Verification items for the finished model (mm, model axes). Coordinates: 2 decimals unless noted, no trailing zeros. Write each loop counter-clockwise with the first axis right and the second up, starting at its lowest first coordinate (ties: lowest second). Pieces come first, ordered by that corner, then holes. Notation, with made-up numbers: M 60.25,0.5 L 81.25,0.5 A12 ccw 81.25,19.5 Z; hole C 79.25,35.5 d11. An arc over 180 degrees is marked long. Answer in a Markdown table with one row per item.
Autodesk Fusion 360 part; units mm, degrees
sketch "スケッチ1" plane through (0, 0, 0) normal (0, 1, 0) x (1, 0, 0)
  line L0 (-132, 0) -> (132, 0)
  line L1 (-132, 0) -> (-132, -10)
  line L2 (-132, -10) -> (-128, -10)
  line L3 (-128, -10) -> (-128, -20)
  line L4 (-128, -20) -> (-132, -20)
  line L5 (-132, -20) -> (-132, -30)
  line L6 (-132, -30) -> (-128, -30)
  line L7 (-128, -30) -> (-128, -40)
  line L8 (-128, -40) -> (-132, -40)
  line L9 (-132, -40) -> (-132, -50)
  line L10 (-132, -50) -> (-77, -50)
  line L11 (-77, -50) -> (-77, -42)
  line L12 (132, 0) -> (132, -10)
  line L13 (132, -10) -> (128, -10)
  line L14 (128, -10) -> (128, -20)
  line L15 (128, -20) -> (132, -20)
  line L16 (132, -20) -> (132, -30)
  line L17 (132, -30) -> (128, -30)
  line L18 (128, -30) -> (128, -40)
  line L19 (128, -40) -> (132, -40)
  line L20 (132, -40) -> (132, -50)
  line L21 (132, -50) -> (72, -50)
  line L22 (72, -50) -> (72, -42)
  line L23 (-77, -42) -> (-65, -42)
  line L24 (-65, -42) -> (-65, -50)
  line L25 (-37, -50) -> (60, -50)
  line L26 (60, -50) -> (60, -42)
  line L27 (60, -42) -> (72, -42)
  line L28 (-113, -50) -> (-97, -50)
  line L29 (-97, -50) -> (-97, -55)
  line L30 (-97, -55) -> (-113, -55)
  line L31 (-113, -55) -> (-113, -50)
  line L32 (97, -50) -> (113, -50)
  line L33 (113, -50) -> (113, -55)
  line L34 (113, -55) -> (97, -55)
  line L35 (97, -55) -> (97, -50)
  line L36 (-38, 0) -> (38, 0)
  line L37 (38, 0) -> (38, -12)
  line L38 (38, -12) -> (-38, -12)
  line L39 (-38, -12) -> (-38, 0)
  line L40 (-37, -50) -> (-37, -42)
  line L41 (-37, -42) -> (-55, -42)
  line L42 (-55, -42) -> (-55, -50)
  line L43 (-55, -50) -> (-65, -50)
  point P0 (0, -20)
  point P1 (-105, -50)
  point P2 (105, -50)
  dimension "d1" = 264
  dimension "d2" = 10
  dimension "d3" = 10
  dimension "d4" = 10
  dimension "d5" = 10
  dimension "d6" = 10
  dimension "d7" = 4
  dimension "d8" = 55
  dimension "d9" = 4
  dimension "d10" = 60
  dimension "d11" = 8
  dimension "d28" = 12
  dimension "d40" = 16
  dimension "d41" = 5
  dimension "d42" = 105
  dimension "d43" = 105
  dimension "d48" = 12
  dimension "d62" = 12
  dimension "d63" = 76
  dimension "d64" = 10
  dimension "d65" = 18
extrude "押し出し1" add sketch "スケッチ1" along normal blind 4 contours L0 L1 L2 L3 L4 L5 L6 L7 L8 L9 L10 L11 L12 L13 L14 L15 L16 L17 L18 L19 L20 L21 L22 L23 L24 L25 L26 L27 L28 L32 L37 L38 L39 L40 L41 L42 L43 | L10 L28 L29 L30 L31 | L21 L32 L33 L34 L35
sketch "スケッチ2" plane through (0, 4, 0) normal (0, 1, 0) x (-1, 0, 0)
  line L0 (-72, 42) -> (-72, 50)
  line L1 (-72, 50) -> (-97, 50)
  line L2 (-132, 50) -> (-132, 40)
  line L3 (-132, 40) -> (-128, 40)
  line L4 (-128, 40) -> (-128, 30)
  line L5 (-128, 30) -> (-132, 30)
  line L6 (-132, 30) -> (-132, 20)
  line L7 (-132, 20) -> (-128, 20)
  line L8 (-128, 20) -> (-128, 10)
  line L9 (-128, 10) -> (-132, 10)
  line L10 (-132, 10) -> (-132, 0)
  line L11 (38, 0) -> (132, 0)
  line L12 (65, 5) -> (-65, 5)
  line L13 (123, 25) -> (-123, 25)
  line L14 (105, 36.5) -> (-105, 36.5)
  line L15 (37, 50) -> (-60, 50)
  line L16 (-60, 50) -> (-60, 42)
  line L17 (-60, 42) -> (-72, 42)
  line L18 (132, 0) -> (132, 10)
  line L19 (132, 10) -> (128, 10)
  line L20 (128, 10) -> (128, 20)
  line L21 (128, 20) -> (132, 20)
  line L22 (132, 20) -> (132, 30)
  line L23 (132, 30) -> (128, 30)
  line L24 (128, 30) -> (128, 40)
  line L25 (128, 40) -> (132, 40)
  line L26 (132, 40) -> (132, 50)
  line L27 (132, 50) -> (113, 50)
  line L28 (77, 50) -> (77, 42)
  line L29 (77, 42) -> (65, 42)
  line L30 (65, 42) -> (65, 50)
  line L31 (113, 50) -> (113, 55)
  line L32 (113, 55) -> (97, 55)
  line L33 (97, 55) -> (97, 50)
  line L34 (97, 50) -> (77, 50)
  line L35 (-97, 50) -> (-97, 55)
  line L36 (-97, 55) -> (-113, 55)
  line L37 (-113, 55) -> (-113, 50)
  line L38 (-113, 50) -> (-132, 50)
  line L39 (-38, 0) -> (-38, 12)
  line L40 (-38, 12) -> (38, 12)
  line L41 (38, 12) -> (38, 0)
  line L42 (-132, 0) -> (-38, 0)
  line L43 (65, 50) -> (55, 50)
  line L44 (55, 50) -> (55, 42)
  line L45 (55, 42) -> (37, 42)
  line L46 (37, 42) -> (37, 50)
  dimension "d14" = 5
  dimension "d15" = 65
  dimension "d16" = 65
  dimension "d17" = 25
  dimension "d19" = 5
  dimension "d24" = 105
  dimension "d25" = 105
  dimension "d46" = 13.5
  dimension "d47" = 5
hole "穴1" at (-65, 4, 5) at (-123, 4, 25) at (65, 4, 5) at (123, 4, 25) at (-105, 4, 36.5) at (105, 4, 36.5) direction (0, -1, 0) diameter 3.2 end through all
sketch "スケッチ3" plane through (0, 4, 0) normal (0, 1, 0) x (-1, 0, 0)
  circle A0 centre (-65, 5) radius 1.6
  circle A1 centre (123, 25) radius 1.6
  circle A2 centre (-123, 25) radius 1.6
  circle A3 centre (-105, 36.5) radius 1.6
  line L0 (132, 0) -> (132, 10)
  line L1 (132, 10) -> (128, 10)
  line L2 (128, 10) -> (128, 20)
  line L3 (128, 20) -> (132, 20)
  line L4 (132, 20) -> (132, 30)
  line L5 (132, 30) -> (128, 30)
  line L6 (128, 30) -> (128, 40)
  line L7 (128, 40) -> (132, 40)
  line L8 (132, 40) -> (132, 50)
  line L9 (132, 50) -> (113, 50)
  line L10 (77, 50) -> (77, 42)
  line L11 (77, 42) -> (65, 42)
  line L12 (65, 42) -> (65, 50)
  line L13 (37, 50) -> (-60, 50)
  line L14 (-60, 50) -> (-60, 42)
  line L15 (-60, 42) -> (-72, 42)
  line L16 (-72, 42) -> (-72, 50)
  line L17 (-72, 50) -> (-97, 50)
  line L18 (-132, 50) -> (-132, 40)
  line L19 (-132, 40) -> (-128, 40)
  line L20 (-128, 40) -> (-128, 30)
  line L21 (-128, 30) -> (-132, 30)
  line L22 (-132, 30) -> (-132, 20)
  line L23 (-132, 20) -> (-128, 20)
  line L24 (-128, 20) -> (-128, 10)
  line L25 (-128, 10) -> (-132, 10)
  line L26 (-132, 10) -> (-132, 0)
  line L27 (38, 0) -> (132, 0)
  circle A4 centre (-108, 15) radius 4.5
  circle A5 centre (-83, 25) radius 15
  line L28 (-83, 8) -> (-83, 42)
  line L29 (113, 50) -> (113, 55)
  line L30 (113, 55) -> (97, 55)
  line L31 (97, 55) -> (97, 50)
  line L32 (97, 50) -> (77, 50)
  line L33 (-97, 50) -> (-97, 55)
  line L34 (-97, 55) -> (-113, 55)
  line L35 (-113, 55) -> (-113, 50)
  line L36 (-113, 50) -> (-132, 50)
  line L37 (75, 9) -> (95.5, 9)
  line L38 (95.5, 9) -> (95.5, 32)
  line L39 (95.5, 32) -> (75, 32)
  line L40 (75, 32) -> (75, 9)
  line L41 (75, 9) -> (95.5, 32) construction
  line L42 (95.5, 9) -> (75, 32) construction
  line L43 (78.25, 6.1) -> (92.25, 6.1)
  line L44 (92.25, 6.1) -> (92.25, 10.1)
  line L45 (92.25, 10.1) -> (78.25, 10.1)
  line L46 (78.25, 10.1) -> (78.25, 6.1)
  line L47 (78.25, 6.1) -> (92.25, 10.1) construction
  line L48 (92.25, 6.1) -> (78.25, 10.1) construction
  line L49 (-38, 0) -> (-38, 12)
  line L50 (-38, 12) -> (38, 12)
  line L51 (38, 12) -> (38, 0)
  line L52 (-132, 0) -> (-38, 0)
  line L53 (65, 50) -> (55, 50)
  line L54 (55, 50) -> (55, 42)
  line L55 (55, 42) -> (37, 42)
  line L56 (37, 42) -> (37, 50)
  point P0 (85.25, 20.5)
  point P1 (85.25, 8.1)
  dimension "d29" = 34
  dimension "d30" = 30
  dimension "d31" = 9
  dimension "d32" = 15
  dimension "d33" = 20
  dimension "d34" = 25
  dimension "d35" = 45
  dimension "d51" = 23
  dimension "d52" = 20.5
  dimension "d53" = 4
  dimension "d54" = 14
  dimension "d55" = 12.4
  dimension "d56" = 75
  dimension "d57" = 9
extrude "押し出し2" cut sketch "スケッチ3" against normal through all contours A4
hole "穴2" at (83, 4, 42) at (83, 4, 8) direction (0, -1, 0) diameter 2.3 depth 35 tip angle 118
extrude "押し出し3" cut sketch "スケッチ3" against normal through all contours L37 L44 L45 L46 | L37 L43 L44 L46
hole "穴3" at (0, 0, 0) at (-75, 4, 9) at (-75, 4, 32) at (-95.5, 4, 32) direction (0, -1, 0) diameter 3.2 depth 16 tip angle 118
1) Sectioned sample at A-A (x = -81.5). Record the cut outline in (y, z), then the cut area to 3 significant figures.
Response values:
| item | result |
|---|---|
| outline | M 0,0 L 4,0 L 4,6.1 L 0,6.1 Z; M 0,10.1 L 4,10.1 L 4,50 L 0,50 Z |
| area | 184 mm² |
2) Thickness scan on L1, parallel to X at y = 2, z = 32; L2, parallel to X at y = 1.6, z = 5; L3, parallel to Z at x = 83, y = 2.3. Record the ranges inside material, lowest first. Write a range as [from, to].
Response values:
| item | result |
|---|---|
| L1 | x = [-128, -97.1], [-93.9, -76.6], [-73.4, 128] |
| L2 | x = [-132, -66.6], [-63.4, -38], [38, 63.4], [66.6, 132] |
| L3 | z = [0, 6.85], [9.15, 40.85], [43.15, 50] |
3) Sectioned sample at B-B (y = 3.3). Give the number of separate pieces and of enclosed holes in the cut face, then the cut area to 3 significant figures.
Response values:
| item | result |
|---|---|
| separate pieces | 1 |
| enclosed holes | 13 |
| area | 11,800 mm² |
4) Release check for a two-part mould opening along X. For faces 1 (the face through (112.496, 2.028, 15.198)), 2 (the face through (-2, 0, 27)) record: +X half, -X half, draft (parallel to the pull), parting line (faces both ways), or undercut.
Response values:
| item | result |
|---|---|
| face 1 | undercut |
| face 2 | draft |
5) Sectioned sample at C-C (x = 75.5). Record the cut outline in (y, z).
Response values:
| item | result |
|---|---|
| outline | M 0,0 L 4,0 L 4,50 L 0,50 Z |
6) Depth check by flat-ended pin: pin 1 (2 mm diameter, centred on x = -124, y = 2, fed in from +Z); pin 2 (2 mm diameter, centred on x = -82.5, y = 1.5, fed in from -Z). Enter the tip coordinate at first touch or a pass-through.
Response values:
| item | result |
|---|---|
| pin 1 | stops at z = 50 |
| pin 2 | stops at z = 0 |
